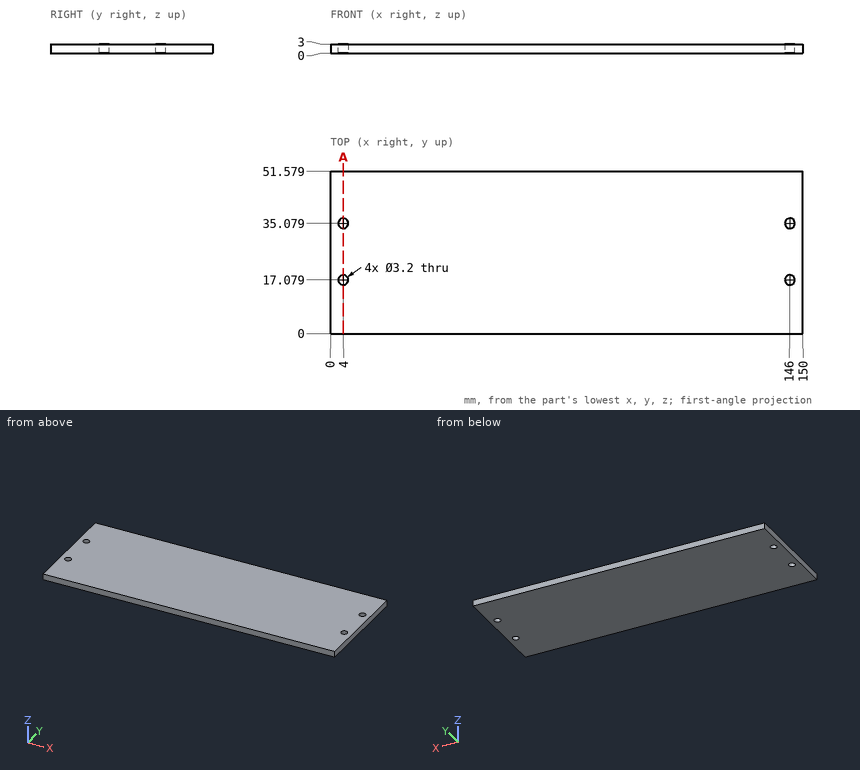
Print and shaded views of the part. All mm, measured from the part's lowest x, y and z. Round coordinates to 2 decimals unless told otherwise and drop trailing zeros. Order: outer loops, then holes, each group sorted by start corner. A loop starts at its lowest first (then second) coordinate and runs counter-clockwise, first axis right, second up.
Q1. Slice it at A-A (x = 4). Write the cut outline in (y, z).
Q2. Drop a flat-ended pin along its axis: pin 1 (8 mm diameter, centred on x = 117.5, y = 6, fed in from -Z). Give the stop position or say it passes through.
Q3. Wall check: L1, parallel to X at y = 35, z = 2.25; L2, parallel to Y at x = 146, z = 1.9; L3, parallel to X at y = 36.5, z = 0.7 (1 decimal). Give the ranges that are in metal, low to high.
Results below:
1. outline: (0, 0) - (15.48, 0) - (15.48, 3) - (0, 3) - close; (18.68, 0) - (33.48, 0) - (33.48, 3) - (18.68, 3) - close; (36.68, 0) - (51.58, 0) - (51.58, 3) - (36.68, 3) - close
2. pin 1: stops at z = 0
3. L1: x = 0 to 2.4, 5.6 to 144.4, 147.6 to 150
3. L2: y = 0 to 15.48, 18.68 to 33.48, 36.68 to 51.58
3. L3: x = 0 to 3.3, 4.7 to 145.3, 146.7 to 150
